Read the model definition and answer for the solid it produces. Units are mm, in the model's axes. A direction names the side the tool comes from. Round coordinates to 2 decimals unless told otherwise and drop trailing zeros. Loops run counter-clockwise (first coordinate to the right, second up) from the corner with the lowest first, then second, coordinate; pieces in that order, holes last. Notation, with made-up numbers: (28.5, 86) -> (81.5, 86) arc R18 ccw to (81.5, 94) -> close; hole circle Ø6 at (-2.75, 31). An arc over 180 degrees is marked (long way). Put each result on its own line as item: value.
from build123d import *

# Parameters (mm, degrees)
BOSS_EXTRUDE1_DEPTH = 3.175
CUT_EXTRUDE1_DEPTH  = 13.131311759


with BuildPart() as part:
    # Sketch1 → Boss-Extrude1 (new body)
    with BuildSketch(Plane.XY):
        Polygon((-10, 2.915), (-10, -2.915), (-8.5, -2.915), (-8.5, -6.09), (-3.5, -6.09), (-3.5, -2.915), (3.5, -2.915), (3.5, -6.09), (8.5, -6.09), (8.5, -2.915), (10, -2.915), (10, 2.915), (8.5, 2.915), (8.5, 6.09), (3.5, 6.09), (3.5, 2.915), (-3.5, 2.915), (-3.5, 6.09), (-8.5, 6.09), (-8.5, 2.915), align=None)
    extrude(amount=BOSS_EXTRUDE1_DEPTH)

    # Sketch2 → Cut-Extrude1 (cut, through all)
    with BuildSketch(Plane.XY.offset(3.175)):
        Polygon((-1.5, 2.915), (-1.5, 1.415), (-3.05, 1.415), (-3.05, -0.985), (-1.5, -0.985), (-1.5, -1.41), (1.5, -1.41), (1.5, -0.985), (3.05, -0.985), (3.05, 1.415), (1.5, 1.415), (1.5, 2.915), align=None)
    extrude(amount=-CUT_EXTRUDE1_DEPTH, mode=Mode.SUBTRACT)


solid = part.part
Item 1: For a pull along X with two mould halves and no side action, classify faces 1 (the flat face through (8.5, 4, 2)), 2 (the flat face through (-9, -2.915, 2)), 3 (the flat face through (2, 1.415, 2)) as pulls with the +X half, pulls with the -X half, needs draft (parallel to the pull), parting line crosses it, or undercut.
Derived:
face 1: pulls with the +X half
face 2: needs draft
face 3: undercut
Item 2: The part is cut by section A-A (y = -3.25). Determine the outline of the cut face in (x, z) (3 decimals), then the cut area to 4 significant figures.
Derived:
outline: (-8.5, 0) -> (-3.5, 0) -> (-3.5, 3.175) -> (-8.5, 3.175) -> close; (3.5, 0) -> (8.5, 0) -> (8.5, 3.175) -> (3.5, 3.175) -> close
area: 31.75 mm^2
Item 3: Flat-ended cylindrical pins translate along their axes: pin 1 Ø1 at (y, z) = (5, 2) entering from +X; pin 2 Ø1.6 at (x, z) = (0.5, 1.5) entering from -Y (3 decimals); pin 3 Ø1.2 at (x, z) = (-9.5, 1) entering from +Y (3 decimals). Find the tip coordinate at first contact, or state that the pin passes through.
Derived:
pin 1: stops at x = 8.5
pin 2: stops at y = -2.915
pin 3: stops at y = 2.915
Item 4: Which of the six approach directions +Z, -Z, +X, -X, +Y, -Y give full straight-line access (tool end or side, diameter ignored) to faces 4 (the flat face through (-9, 2.915, 2)), 5 (the flat face through (3.5, -4, 2)), 6 (the flat face through (1.5, 2, 2)), 7 (the flat face through (-2.4, -1.3, 3.175)), 8 (the flat face through (-2, -0.985, 2))?
Derived:
face 4: +Z, -Z, -X, +Y
face 5: +Z, -Z, -Y
face 6: +Z, -Z, +Y
face 7: +Z, +X, -X, +Y, -Y
face 8: +Z, -Z
Item 5: The part is cut by section B-B (x = 2.25). Determine the outline of the cut face in (y, z) (3 decimals).
Derived:
outline: (-2.915, 0) -> (-0.985, 0) -> (-0.985, 3.175) -> (-2.915, 3.175) -> close; (1.415, 0) -> (2.915, 0) -> (2.915, 3.175) -> (1.415, 3.175) -> close
Item 6: Find the intervals of material crossed by line 1 along X through (y, z) = (3, 2.1); line 2 along X through (y, z) = (2, 1.95); line 3 along Y through (x, z) = (-2, 2.95) (3 decimals), in increasing order.
Derived:
line 1: x = -8.5 to -3.5, 3.5 to 8.5
line 2: x = -10 to -1.5, 1.5 to 10
line 3: y = -2.915 to -0.985, 1.415 to 2.915
